```python
from build123d import *

# Parameters (mm, degrees)
PAD_DEPTH         = 4
SKETCH003_W       = 90
SKETCH003_H       = 4
PAD001_DEPTH      = 54
SKETCH002_W       = 5
SKETCH002_H       = 4
PAD002_DEPTH      = 51
SKETCH006_R       = 2
POCKET_DEPTH      = 84.001
POCKET_DEPTH_BACK = 14.001
SKETCH005_W       = 70
SKETCH005_H       = 1.5
PAD003_DEPTH      = 10
SKETCH004_W       = 1.5
SKETCH004_H       = 3
SKETCH004_W_2     = 2.5
SKETCH004_H_2     = 0.9
PAD004_DEPTH      = 46.5
SKETCH_R          = 2.5
PAD005_DEPTH      = 10
POCKET001_START   = 4
SKETCH007_R       = 1.5
POCKET001_DEPTH   = 20


with BuildPart() as part:
    # Sketch001 → Pad (new body)
    with BuildSketch(Plane.XY):
        with BuildLine():
            Line((0, 94), (0, 5))
            ThreePointArc((0, 5), (1.464466, 1.464466), (5, 0))
            Line((5, 0), (85, 0))
            ThreePointArc((85, 0), (88.535534, 1.464466), (90, 5))
            Line((90, 5), (90, 94))
            Line((90, 94), (0, 94))
        make_face()
    extrude(amount=PAD_DEPTH)

    # Sketch003 → Pad001 (join)
    with BuildSketch(Plane.XY):
        with Locations((45, 96)):
            Rectangle(SKETCH003_W, SKETCH003_H)
    extrude(amount=PAD001_DEPTH)

    # Sketch002 → Pad002 (join)
    with BuildSketch(Plane.XY):
        with Locations((17.5, 92)):
            Rectangle(SKETCH002_W, SKETCH002_H)
        with Locations((17.5, 24)):
            Rectangle(SKETCH002_W, SKETCH002_H)
        with Locations((23.7, 92)):
            Rectangle(SKETCH002_W, SKETCH002_H)
        with Locations((23.7, 24)):
            Rectangle(SKETCH002_W, SKETCH002_H)
    extrude(amount=PAD002_DEPTH)

    # Sketch006 → Pocket (cut, two sides)
    with BuildSketch(Plane(origin=(0, 84, 0), x_dir=(-1, 0, 0), z_dir=(0, 1, 0))) as pocket_sk:
        with Locations((-30, 25)):
            Circle(SKETCH006_R)
        with Locations((-60, 25)):
            Circle(SKETCH006_R)
    extrude(amount=-POCKET_DEPTH, mode=Mode.SUBTRACT)
    extrude(pocket_sk.sketch, amount=POCKET_DEPTH_BACK, mode=Mode.SUBTRACT)

    # Sketch005 → Pad003 (join)
    with BuildSketch(Plane.XY):
        with Locations((45, 1.75)):
            Rectangle(SKETCH005_W, SKETCH005_H)
    extrude(amount=PAD003_DEPTH)

    # Sketch004 → Pad004 (join)
    with BuildSketch(Plane.XY):
        with Locations((2.25, 92.5)):
            Rectangle(SKETCH004_W, SKETCH004_H)
        with Locations((2.25, 90.55)):
            Rectangle(SKETCH004_W_2, SKETCH004_H_2)
        with Locations((87.75, 92.5)):
            Rectangle(SKETCH004_W, SKETCH004_H)
        with Locations((87.75, 90.55)):
            Rectangle(SKETCH004_W_2, SKETCH004_H_2)
    extrude(amount=PAD004_DEPTH)

    # Sketch → Pad005 (join)
    with BuildSketch(Plane.XY):
        with Locations((80, 50)):
            Circle(SKETCH_R)
        with Locations((80, 23)):
            Circle(SKETCH_R)
        with Locations((50, 50)):
            Circle(SKETCH_R)
        with Locations((50, 23)):
            Circle(SKETCH_R)
    extrude(amount=PAD005_DEPTH)

    # Sketch007 → Pocket001 (cut)
    with BuildSketch(Plane.XY.offset(POCKET001_START)):
        with Locations((80, 50)):
            Circle(SKETCH007_R)
        with Locations((80, 23)):
            Circle(SKETCH007_R)
        with Locations((50, 50)):
            Circle(SKETCH007_R)
        with Locations((50, 23)):
            Circle(SKETCH007_R)
    extrude(amount=POCKET001_DEPTH, mode=Mode.SUBTRACT)


solid = part.part
```
For this review, take the finished solid that the model builds, in its own axes (mm). A direction names the side the tool comes from. Round coordinates to 2 decimals unless told otherwise and drop trailing zeros. Loops run counter-clockwise (first coordinate to the right, second up) from the corner with the lowest first, then second, coordinate; pieces in that order, holes last.
(1) Tool access review of faces 5 (the cylindrical face through (28.153, 95.972, 24.234)), 6 (the flat face through (0, 65, 3)), 7 (the flat face through (24, 90, 27)), 8 (the flat face through (50, 48, 10)), 9 (the flat face through (88, 92, 46.5)): name each direction out of +Z, -Z, +X, -X, +Y, -Y from which nothing blocks a thin tool from reaching the whole face with its end or side.
Returned:
face 5: +Y, -Y
face 6: +Z, -Z, -X, +Y, -Y
face 7: +Z, +X, -X
face 8: +Z, +X, -X, -Y
face 9: +Z, +X, -Y
(2) Clearance check with flat-ended pins moving along their axes: P1, Ø0.9, axis at y = 93, z = 14.5, coming from the -X side; P2, Ø4.5, axis at x = 23.5, y = 23.5, coming from the +Z side; P3, Ø2, axis at y = 24.5, z = 17.5, coming from the -X side. State where each tip first meets the part, or that it passes through.
Returned:
P1: stops at x = 1.5
P2: stops at z = 51
P3: stops at x = 15
(3) Wall thickness on line 1 along X through (y, z) = (23, 5); line 2 along Y through (x, z) = (50, 8.65); line 3 along X through (y, z) = (95.65, 25): over which ranges is each line inside the solid? List them lowest first.
Returned:
line 1: x = 15 to 20, 21.2 to 26.2, 47.5 to 48.5, 51.5 to 52.5, 77.5 to 78.5, 81.5 to 82.5
line 2: y = 1 to 2.5, 20.5 to 21.5, 24.5 to 25.5, 47.5 to 48.5, 51.5 to 52.5, 94 to 98
line 3: x = 0 to 28, 32 to 58, 62 to 90
(4) Mouldability with a two-part tool opening along Y and no side actions: class faces 1 (the cylindrical face through (48.89, 24.01, 6.96)), 2 (the flat face through (17, 92, 51)), 3 (the flat face through (45, 1, 7)), 4 (the flat face through (45, 2.5, 7)) as released by +Y, released by -Y, zero draft, split by the parting line, or undercut.
Returned:
face 1: undercut
face 2: zero draft
face 3: released by -Y
face 4: undercut
(5) We need section A-A (x = 60). Give the boundary of the cut face in (y, z), plus the area to 3 significant figures.
Returned:
outline: (0, 0) - (98, 0) - (98, 23) - (94, 23) - (94, 4) - (2.5, 4) - (2.5, 10) - (1, 10) - (1, 4) - (0, 4) - close; (94, 27) - (98, 27) - (98, 54) - (94, 54) - close
area: 585 mm2
(6) We need section D-D (y = 78.5). Give the boundary of the cut face in (x, z).
Returned:
outline: (0, 0) - (90, 0) - (90, 4) - (0, 4) - close
(7) We need section C-C (z = 29). State how many separate pieces and enclosed holes the cut face has, plus the area to 4 significant figures.
Returned:
separate pieces: 3
enclosed holes: 0
area: 453.5 mm2
(8) We need section B-B (x = 50). Give the boundary of the cut face in (y, z).
Returned:
outline: (0, 0) - (98, 0) - (98, 54) - (94, 54) - (94, 4) - (52.5, 4) - (52.5, 10) - (51.5, 10) - (51.5, 4) - (48.5, 4) - (48.5, 10) - (47.5, 10) - (47.5, 4) - (25.5, 4) - (25.5, 10) - (24.5, 10) - (24.5, 4) - (21.5, 4) - (21.5, 10) - (20.5, 10) - (20.5, 4) - (2.5, 4) - (2.5, 10) - (1, 10) - (1, 4) - (0, 4) - close
